Can you work these out from the drawing? Everything is in mm from the part's minimum corner. A direction names the side the tool comes from. Give positions to 0.01 mm unless a question says otherwise; leave off trailing zeros. Order: outer loops, then holes, each group sorted by start corner. A loop starts at its lowest first (then second) coordinate and runs counter-clockwise, first axis right, second up. Notation, with made-up numbers: M 64.25,0.5 L 101.25,0.5 A32 ccw 101.25,26.5 Z; hole C 48.5,19 d6. An arc over 180 degrees is marked long. Answer in a Markdown table with one row per item. Add a question column.
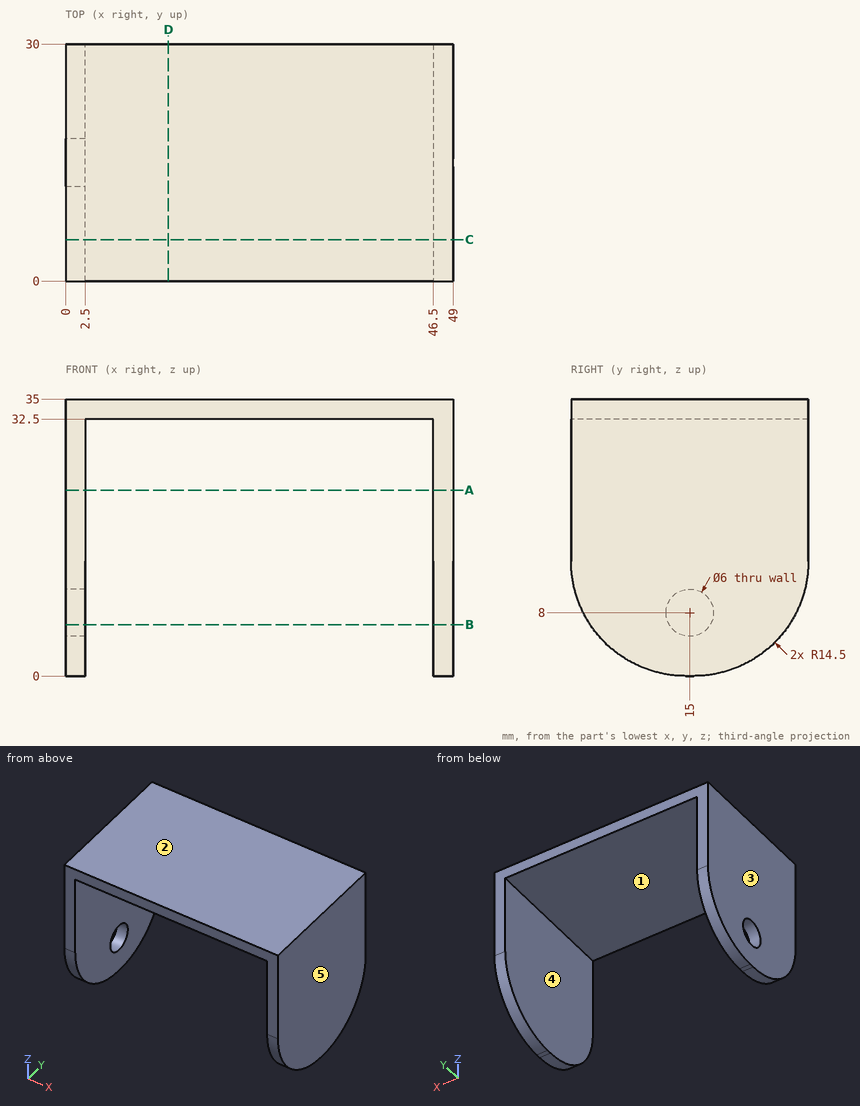
1. Will these pins go through, and if not, where does the flat tip stop? P1, Ø1.5, axis at x = 39.5, y = 15.5, coming from the -Z side; P2, Ø5.5, axis at y = 15, z = 8, coming from the -X side; P3, Ø5, axis at x = 12.5, z = 30.5, coming from the +Y side.
2. Suppose I cut it at C-C on y = 5.25. List the corners of the cut face in (x, z) for me.
3. Suppose I cut it at B-B on z = 6.5. List the corners of the cut face in (x, y) for me.
4. Suppose I cut it at A-A on z = 23.5. List the corners of the cut face in (x, y) for me.
5. Thinking about a two-plate mould opening in X: for the marked faces 1, 2 and 3, which applies, pulls with the +X half, pulls with the -X half, needs draft (parallel to the pull), parting line crosses it, or undercut?
6. Suppose I cut it at D-D on x = 13. List the corners of the cut face in (y, z) for me, plus the area to 3 significant figures.
7. If I drill on line 1 along X through (y, z) = (5.25, 7); line 2 along Z through (x, y) = (1.9, 15); line 3 along Z through (x, y) = (41.5, 2), over which ranges is the centre line in solid material (lowest first)? Write a range as [from, to].
8. For the marked faces 4 and 5, which set-ups out of +Z, -Z, +X, -X, +Y, -Y let a thin tool reach every point of the face, with its end or its side?
Findings below:
| question | item | result |
|---|---|---|
| 1 | P1 | z = 32.5 |
| 1 | P2 | x = 46.5 |
| 1 | P3 | y = 30 |
| 2 | outline | M 0,3.33 L 2.5,3.33 L 2.5,32.5 L 46.5,32.5 L 46.5,3.33 L 49,3.33 L 49,35 L 0,35 Z |
| 3 | outline | M 0,2.41 L 2.5,2.41 L 2.5,12.4 L 0,12.4 Z; M 0,17.6 L 2.5,17.6 L 2.5,27.59 L 0,27.59 Z; M 46.5,2.41 L 49,2.41 L 49,27.59 L 46.5,27.59 Z |
| 4 | outline | M 0,0 L 2.5,0 L 2.5,30 L 0,30 Z; M 46.5,0 L 49,0 L 49,30 L 46.5,30 Z |
| 5 | face 1 | undercut |
| 5 | face 2 | needs draft |
| 5 | face 3 | pulls with the -X half |
| 6 | outline | M 0,32.5 L 30,32.5 L 30,35 L 0,35 Z |
| 6 | area | 75.0 mm2 |
| 7 | line 1 | [0, 2.5], [46.5, 49] |
| 7 | line 2 | [0, 5], [11, 35] |
| 7 | line 3 | [32.5, 35] |
| 8 | face 4 | -Z, +Y, -Y |
| 8 | face 5 | +Z, -Z, +X, +Y, -Y |
